Check sheet for the drawn part. Datum: minimum x, y, z corner. Units: mm. A direction names the side the tool comes from. Coordinates: 2 decimals unless noted, no trailing zeros. Loops run counter-clockwise (first coordinate to the right, second up) from the corner with the lowest first, then second, coordinate; pieces in that order, holes last.
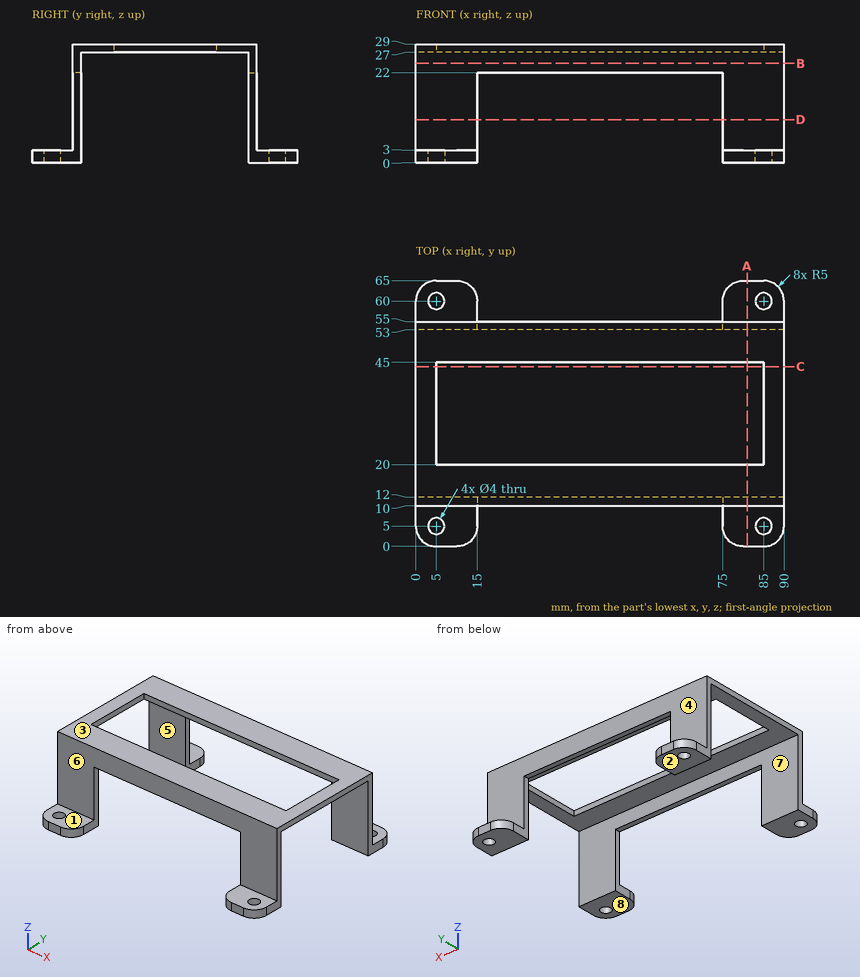
1) Depth check by flat-ended pin: pin 1 (11 mm diameter, centred on x = 5, y = 61, fed in from +Z); pin 2 (1.5 mm diameter, centred on y = 56, z = 11.5, fed in from +X); pin 3 (5 mm diameter, centred on y = 11, z = 15.5, fed in from -X); pin 4 (0.6 mm diameter, centred on x = 31.5, y = 54, fed in from -Z). Enter the tip coordinate at first touch or a pass-through.
Answer sheet:
pin 1: stops at z = 3
pin 2: passes through
pin 3: stops at x = 0
pin 4: stops at z = 22
2) Section check D-D on z = 10.5. Enter the section's corners in (x, y), plus the area to 3 significant figures.
Answer sheet:
outline: (0, 10) - (15, 10) - (15, 12) - (0, 12) - close; (0, 53) - (15, 53) - (15, 55) - (0, 55) - close; (75, 10) - (90, 10) - (90, 12) - (75, 12) - close; (75, 53) - (90, 53) - (90, 55) - (75, 55) - close
area: 120 mm2
3) Section check A-A on x = 81. Enter the section's corners in (y, z).
Answer sheet:
outline: (0, 0) - (12, 0) - (12, 27) - (20, 27) - (20, 29) - (10, 29) - (10, 3) - (0, 3) - close; (45, 27) - (53, 27) - (53, 0) - (65, 0) - (65, 3) - (55, 3) - (55, 29) - (45, 29) - close
4) Mould release check, pull along Y, two halves, no side actions. Record for the marked faces 6, 7 and 8: +Y half, -Y half, draft (parallel to the pull), parting line (faces both ways), or undercut.
Answer sheet:
face 6: -Y half
face 7: undercut
face 8: draft
5) Set-up check for the marked faces 1, 2, 3, 4 and 5: record each of +Z, -Z, +X, -X, +Y, -Y from which the full face is reachable in a straight line by a thin tool's end or side.
Answer sheet:
face 1: +Z, +X, -X, -Y
face 2: -Z, +X, -X, +Y, -Y
face 3: +Z, +X, -X, +Y, -Y
face 4: +Z, +X, -X, +Y
face 5: -Z, +X, -X
6) Scan lines: line 1 (Y direction, x = 5, z = 1.8); line 2 (X direction, y = 10.5, z = 10.5); line 3 (Z direction, x = 55, y = 45.5). Record each from-to range of solid material in increasing order.
Answer sheet:
line 1: y = 0 to 3, 7 to 12, 53 to 58, 62 to 65
line 2: x = 0 to 15, 75 to 90
line 3: z = 27 to 29
7) Section check B-B on z = 24.25. Enter the section's corners in (x, y).
Answer sheet:
outline: (0, 10) - (90, 10) - (90, 12) - (0, 12) - close; (0, 53) - (90, 53) - (90, 55) - (0, 55) - close
8) Section check C-C on y = 44. Enter the section's corners in (x, z).
Answer sheet:
outline: (0, 27) - (5, 27) - (5, 29) - (0, 29) - close; (85, 27) - (90, 27) - (90, 29) - (85, 29) - close
